Verification items for the finished model (mm, model axes). Round coordinates to 2 decimals unless told otherwise and drop trailing zeros. Order: outer loops, then holes, each group sorted by start corner. A loop starts at its lowest first (then second) coordinate and runs counter-clockwise, first axis right, second up. Notation, with made-up numbers: M 19,-11.5 L 56,-11.5 A22 cw 56,9.5 Z; hole C 57,-33 d4. An arc over 180 degrees is marked long. Return JSON: item names as keys, results as strings. Group by question number.
from build123d import *

# Parameters (mm, degrees)
F0_W     = 38.1
F0_H     = 139.7
F1_DEPTH = 1828.8
F3_DEPTH = 38.101


with BuildPart() as f1:
    # F0 (on Front) → F1 (new body)
    with BuildSketch(Plane.XZ):
        with Locations((19.05, 69.85)):
            Rectangle(F0_W, F0_H)
    extrude(amount=F1_DEPTH)

    # F2 (on face) → F3 (cut, through all)
    with BuildSketch(Plane.YZ.offset(38.1)):
        Polygon((-1758.95, 0), (-1828.8, 69.85), (-1828.8, 0), align=None)
        Polygon((-1828.8, 139.7), (-1828.8, 69.85), (-1758.95, 139.7), align=None)
        Polygon((0, 0), (0, 69.85), (-69.85, 0), align=None)
        Polygon((0, 69.85), (0, 139.7), (-69.85, 139.7), align=None)
    extrude(amount=-F3_DEPTH, mode=Mode.SUBTRACT)


solid = f1.part
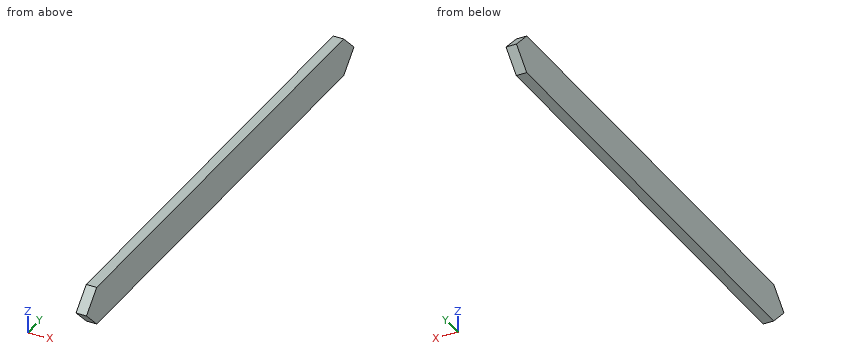
1. Cross-section at A-A (x = 16). Enter the section's corners in (y, z).
2. Cross-section at C-C (z = 122). Enter the section's corners in (x, y), plus the area to 3 significant figures.
3. Cross-section at B-B (z = 42.5). Enter the section's corners in (x, y), plus the area to 3 significant figures.
4. Thickness scan on line 1 along Y through (x, z) = (34, 69.5); line 2 along Y through (x, z) = (7, 117). Record the ranges inside material, lowest first. Write a range as from..to.
5. Go/stop test with flat-tipped pins: pin 1 (12 mm diameter, centred on x = 9.5, z = 45.5, fed in from +Y); pin 2 (3 mm diameter, centred on x = 21, y = -1290.5, fed in from -Z). Record where each tip stops, or that it passes through.
Computed:
{
 "1": {"outline": "M -1828.8,69.85 L -1758.95,0 L -69.85,0 L 0,69.85 L -69.85,139.7 L -1758.95,139.7 Z"},
 "2": {"outline": "M 0,-1776.65 L 38.1,-1776.65 L 38.1,-52.15 L 0,-52.15 Z", "area": "65,700 mm²"},
 "3": {"outline": "M 0,-1801.45 L 38.1,-1801.45 L 38.1,-27.35 L 0,-27.35 Z", "area": "67,600 mm²"},
 "4": {"line 1": "y = -1828.45..-0.35", "line 2": "y = -1781.65..-47.15"},
 "5": {"pin 1": "stops at y = -18.35", "pin 2": "stops at z = 0"}
}
